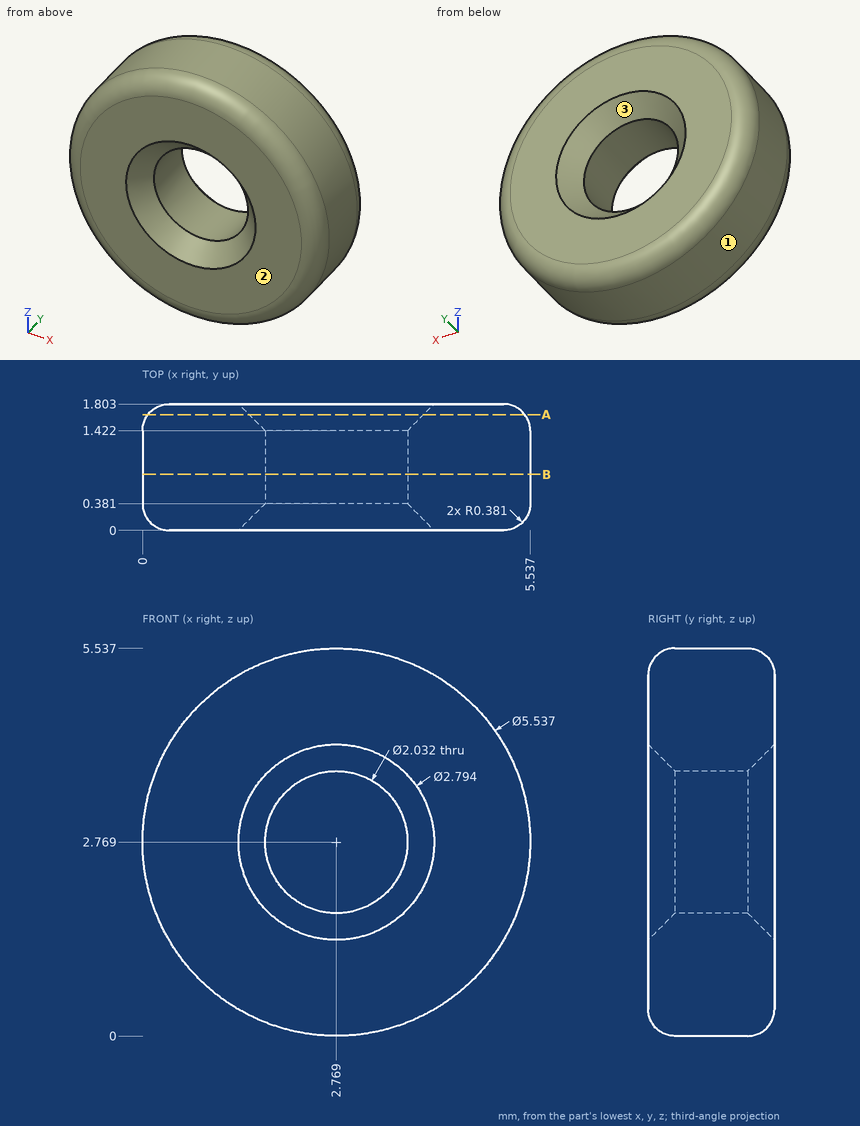
Part print with two shaded views. Sizes in mm from the minimum x, y, z corner. Round coordinates to 2 decimals unless told otherwise and drop trailing zeros. Loops run counter-clockwise (first coordinate to the right, second up) from the corner with the lowest first, then second, coordinate; pieces in that order, holes last.
Item 1: Two-plate mould, pull along X, no slides. Class the marked faces 1, 2 and 3: released by +X, released by -X, zero draft, split by the parting line, or undercut.
Item 2: Drill centre lines: line 1 along Z through (x, y) = (3.35, 0.65) (1 decimal); line 2 along Z through (x, y) = (2.45, 1.5) (1 decimal); line 3 along X through (y, z) = (1.5, 2) (1 decimal). Where is each one in solid material? Low to high.
Item 3: Saw through at A-A (y = 1.65). List the corners of the cut face in (x, z), then the cut area to 3 significant figures.
Item 4: Pin check, flat tips, straight feed: P1, Ø1, axis at y = 0.5, z = 1, coming from the +X side; P2, Ø1.5, axis at x = 3, z = 2.5, coming from the -Y side. Stop position of each tip, or through.
Item 5: Saw through at B-B (y = 0.8). List the corners of the cut face in (x, z) (1 decimal).
Worked answers:
1. face 1: split by the parting line
1. face 2: zero draft
1. face 3: undercut
2. line 1: z = 0.1 to 1.9, 3.6 to 5.5
2. line 2: z = 0 to 1.7, 3.8 to 5.5
2. line 3: x = 0.1 to 2, 3.5 to 5.4
3. outline: circle Ø5.39 at (2.77, 2.77); hole circle Ø2.49 at (2.77, 2.77)
3. area: 17.9 mm2
4. P1: stops at x = 5.23
4. P2: stops at y = 0.29
5. outline: circle Ø5.5 at (2.8, 2.8); hole circle Ø2 at (2.8, 2.8)
